The model under review builds one solid part; all positions refer to its coordinate system, in mm. A direction names the side the tool comes from. Round coordinates to 2 decimals unless told otherwise and drop trailing zeros. Loops run counter-clockwise (first coordinate to the right, second up) from the corner with the lowest first, then second, coordinate; pieces in that order, holes last. Notation, with made-up numbers: M -10,2.5 L 8,2.5 A11 cw 8,19.5 Z; hole C -29.75,4.25 d1. An arc over 180 degrees is marked long. Use a Markdown table: item, result. Add a question column.
```python
from build123d import *

# Parameters (mm, degrees)
SKETCH_1_W            = 162
SKETCH_1_H            = 105
EXTRUDE_1_DEPTH       = 6
CUT_EXTRUDE_1_DEPTH   = 133.747881339
FILLET_1_R            = 1
EXTRUDE_START         = -20
SKETCH_4_W            = 20
SKETCH_4_H            = 14.5
EXTRUDE_2_DEPTH       = 5
F_4_0MM_1_D           = 4
F_4_0MM_1_CSINK_D     = 4.05
F_4_0MM_1_CSINK_ANGLE = 90
EXTRUDE_START_2       = 15
SKETCH_7_W            = 6
SKETCH_7_H            = 9
EXTRUDE_3_DEPTH       = 20.5
SKETCH_8_R            = 1.5
CUT_EXTRUDE_2_DEPTH   = 103.13471496
CUT_EXTRUDE_3_DEPTH   = 134.402586182
EXTRUDE_START_3       = -5
SKETCH_10_W           = 20
SKETCH_10_H           = 14.5
SKETCH_10_R           = 2.025
SKETCH_10_R_2         = 2
EXTRUDE_4_DEPTH       = 5
SKETCH_12_R           = 2.1
SKETCH_12_R_2         = 2.125
SKETCH_12_R_3         = 1.6
CUT_EXTRUDE_4_DEPTH   = 134.402586182


with BuildPart() as part:
    # 草圖1 → 填料-伸長1 (new body)
    with BuildSketch(Plane(origin=(0, 0, 0), x_dir=(1, 0, 0), z_dir=(0, 1, 0))):
        Rectangle(SKETCH_1_W, SKETCH_1_H)
    extrude(amount=EXTRUDE_1_DEPTH)

    # 草圖3 → 除料-伸長1 (cut, through all)
    with BuildSketch(Plane.XY.offset(52.5)):
        with BuildLine():
            Line((75.5, 5), (75.5, 6))
            Line((75.5, 6), (78.5, 6))
            Line((78.5, 6), (78.5, 5))
            ThreePointArc((78.5, 5), (77, 1.677124344), (75.5, 5))
        make_face()
    cut_extrude_1 = extrude(amount=-CUT_EXTRUDE_1_DEPTH, mode=Mode.SUBTRACT)

    # 鏡射1: 除料-伸長1 across plane
    add(cut_extrude_1.mirror(Plane(origin=(0, 0, 0), x_dir=(0, 0, 1), z_dir=(1, 0, 0))), mode=Mode.SUBTRACT)

    # 圓角1
    fillet_1_edges = [part.edges().sort_by_distance(p)[0] for p in [
        (81, 0, 0),
        (-81, 0, 0),
    ]]
    fillet(fillet_1_edges, radius=FILLET_1_R)

    # 草圖4 → 填料-伸長2 (add)
    with BuildSketch(Plane(origin=(0, 0, -52.5), x_dir=(-1, 0, 0), z_dir=(0, 0, -1)).offset(EXTRUDE_START)):
        with Locations((0, -7.25)):
            Rectangle(SKETCH_4_W, SKETCH_4_H)
    extrude(amount=-EXTRUDE_2_DEPTH)

    # Ø4.0mm 定位孔1 (through all)
    with Locations(Plane(origin=(0, 0, -32.5), x_dir=(-1, 0, 0), z_dir=(0, 0, -1))):
        with Locations((5, -8), (-5, -8)):
            CounterSinkHole(F_4_0MM_1_D / 2, F_4_0MM_1_CSINK_D / 2, counter_sink_angle=F_4_0MM_1_CSINK_ANGLE)

    # 草圖7 → 填料-伸長3 (add)
    with BuildSketch(Plane.XY.offset(-27.5).offset(EXTRUDE_START_2)):
        with Locations((19.75, -4.5)):
            Rectangle(SKETCH_7_W, SKETCH_7_H)
        with Locations((-19.75, -4.5)):
            Rectangle(SKETCH_7_W, SKETCH_7_H)
    extrude(amount=EXTRUDE_3_DEPTH)

    # 草圖8 → 除料-伸長2 (cut, through all)
    with BuildSketch(Plane.XY.offset(8)):
        with Locations((-19.75, -6)):
            Circle(SKETCH_8_R)
        with Locations((19.75, -6)):
            Circle(SKETCH_8_R)
    extrude(amount=-CUT_EXTRUDE_2_DEPTH, mode=Mode.SUBTRACT)

    # 草圖9 → 除料-伸長3 (cut, through all)
    with BuildSketch(Plane.XY.offset(52.5)):
        with BuildLine():
            Line((-78.65, 6), (-75.35, 6))
            Line((-75.35, 6), (-75.35, 5.05552922))
            ThreePointArc((-75.35, 5.05552922), (-77, 1.527124344), (-78.65, 5.05552922))
            Line((-78.65, 5.05552922), (-78.65, 6))
        make_face()
        with BuildLine():
            Line((78.65, 5.05552922), (78.65, 6))
            Line((78.65, 6), (75.35, 6))
            Line((75.35, 6), (75.35, 5.05552922))
            ThreePointArc((75.35, 5.05552922), (77, 1.527124344), (78.65, 5.05552922))
        make_face()
    extrude(amount=-CUT_EXTRUDE_3_DEPTH, mode=Mode.SUBTRACT)

    # 草圖10 → 填料-伸長4 (add)
    # profile 1 of 2: a face of its own
    with BuildSketch(Plane(origin=(0, 0, -32.5), x_dir=(-1, 0, 0), z_dir=(0, 0, -1)).offset(EXTRUDE_START_3)):
        with Locations((0, -7.25)):
            Rectangle(SKETCH_10_W, SKETCH_10_H)
        with Locations((5, -8)):
            Circle(SKETCH_10_R, mode=Mode.SUBTRACT)
        with Locations((-5, -8)):
            Circle(SKETCH_10_R_2, mode=Mode.SUBTRACT)
    # profile 2 of 2: a face of its own
    with BuildSketch(Plane(origin=(0, 0, -32.5), x_dir=(-1, 0, 0), z_dir=(0, 0, -1)).offset(EXTRUDE_START_3)):
        with Locations((50, -7.25)):
            Rectangle(SKETCH_10_W, SKETCH_10_H)
        with Locations((55, -8)):
            Circle(SKETCH_10_R, mode=Mode.SUBTRACT)
        with Locations((45, -8)):
            Circle(SKETCH_10_R_2, mode=Mode.SUBTRACT)
    extrude(amount=EXTRUDE_4_DEPTH)

    # 草圖12 → 除料-伸長4 (cut, through all)
    with BuildSketch(Plane.XY.offset(52.5)):
        with Locations((-45, -8)):
            Circle(SKETCH_12_R)
        with Locations((-55, -8)):
            Circle(SKETCH_12_R_2)
        with Locations((-19.75, -6)):
            Circle(SKETCH_12_R_3)
        with Locations((-5, -8)):
            Circle(SKETCH_12_R)
        with Locations((5, -8)):
            Circle(SKETCH_12_R)
        with Locations(Location((19.75, -6, 0), (0, 0, 180))):
            Circle(SKETCH_12_R_3)
    extrude(amount=-CUT_EXTRUDE_4_DEPTH, mode=Mode.SUBTRACT)


solid = part.part
```
(1) For faces 5 (the face through (-40, -7, -30)), 6 (the face through (-60, -7, -30)), 7 (the face through (-50, -7, -32.5)), list the 3-axis set-ups (+Z, -Z, +X, -X, +Y, -Y) from which the entire face can be reached by the end or side of a thin tool; tool diameter is ignored.
(2) Draft analysis for pull direction X (two halves, no side actions). For faces 1 (the face through (81, 3, 1)), 2 (the face through (-81, 3, 1)), 3 (the face through (-76.93, 1.53, 0.73)), 4 (the face through (-20, -3, -12.5)), state which applies: released by +X, released by -X, zero draft, split by the parting line, or undercut.
(3) Consider section A-A, the plane x = -55. Give the boundary of the cut face in (y, z) (3 decimals).
(4) Consider section B-B, the plane y = -2.75. Give the boundary of the cut face in (x, z).
(5) Insertion check: pin 1 Ø6 at (x, y) = (-6.5, -9) entering from -Z; pin 2 Ø2.5 at (x, y) = (-45, -8) entering from -Z; pin 3 Ø3 at (x, z) = (-45.5, -22.5) entering from -Y; pin 4 Ø6.5 at (x, y) = (-19, -4) entering from +Z. Each pin has a flat end and moves straight along its axis. Give the tip position at first contact, or say it passes through.
(6) Consider section D-D, the plane x = 5. Give the boundary of the cut face in (y, z), then the cut area to 4 significant figures.
(7) Consider section C-C, the plane z = -3. Give the boundary of the cut face in (x, y).
(8) To check wall thickness, follow probe 1 along X at (y, z) = (3.75, -41.5); probe 2 along X at (y, z) = (2.25, -28); probe 3 along Y at (x, z) = (-45, -31). State the ranges of each line that lie inside material, in increasing order.
Found:
| question | item | result |
|---|---|---|
| 1 | face 5 | +Z, -Z, -Y |
| 1 | face 6 | +Z, -Z, -X, -Y |
| 1 | face 7 | -Z, +X, -X, -Y |
| 2 | face 1 | released by +X |
| 2 | face 2 | released by -X |
| 2 | face 3 | undercut |
| 2 | face 4 | zero draft |
| 3 | outline | M -14.5,-32.5 L -10.125,-32.5 L -10.125,-27.5 L -14.5,-27.5 Z; M -5.875,-32.5 L 0,-32.5 L 0,-52.5 L 6,-52.5 L 6,52.5 L 0,52.5 L 0,-27.5 L -5.875,-27.5 Z |
| 4 | outline | M -60,-32.5 L -40,-32.5 L -40,-27.5 L -60,-27.5 Z; M -22.75,-12.5 L -16.75,-12.5 L -16.75,8 L -22.75,8 Z; M -10,-32.5 L 10,-32.5 L 10,-27.5 L -10,-27.5 Z; M 16.75,-12.5 L 22.75,-12.5 L 22.75,8 L 16.75,8 Z |
| 5 | pin 1 | stops at z = -32.5 |
| 5 | pin 2 | passes through |
| 5 | pin 3 | stops at y = 0 |
| 5 | pin 4 | stops at z = 8 |
| 6 | outline | M -14.5,-32.5 L -10.1,-32.5 L -10.1,-27.5 L -14.5,-27.5 Z; M -5.9,-32.5 L 0,-32.5 L 0,-52.5 L 6,-52.5 L 6,52.5 L 0,52.5 L 0,-27.5 L -5.9,-27.5 Z |
| 6 | area | 681.5 mm^2 |
| 7 | outline | M -81,1 A1 ccw -80,0 L -22.75,0 L -22.75,-9 L -16.75,-9 L -16.75,0 L 16.75,0 L 16.75,-9 L 22.75,-9 L 22.75,0 L 80,0 A1 ccw 81,1 L 81,6 L 78.65,6 L 78.65,5.06 A2.15 cw long 75.35,5.06 L 75.35,6 L -75.35,6 L -75.35,5.06 A2.15 cw long -78.65,5.06 L -78.65,6 L -81,6 Z; hole C -19.75,-6 d3.2; hole C 19.75,-6 d3.2 |
| 8 | probe 1 | x = -81 to -79.15, -74.85 to 74.85, 79.15 to 81 |
| 8 | probe 2 | x = -81 to -78.61, -75.39 to 75.39, 78.61 to 81 |
| 8 | probe 3 | y = -14.5 to -10.1, -5.9 to 6 |
